For this review, take the finished solid that the model builds, in its own axes (mm). Give positions to 0.01 mm unless a question says otherwise; leave off trailing zeros. Loops run counter-clockwise (first coordinate to the right, second up) from the corner with the lowest first, then second, coordinate; pieces in that order, holes last.
```python
from build123d import *

# Parameters (mm, degrees)
SKETCH1_R           = 1.5
BOSS_EXTRUDE1_DEPTH = 3
BOSS_EXTRUDE2_DEPTH = 3
LPATTERN1_COUNT     = 2
LPATTERN1_PITCH     = 25
BOSS_EXTRUDE3_DEPTH = 3
SKETCH1_4_R         = 1.5
BOSS_EXTRUDE4_DEPTH = 15


with BuildPart() as part:
    # Sketch1 → Boss-Extrude1 (new body)
    with BuildSketch(Plane(origin=(0, 0, 0), x_dir=(1, 0, 0), z_dir=(0, 1, 0))):
        Polygon((0, 53.3), (57.3, 53.3), (57.3, 0), (0, 0), (0, 51.3), align=None)
        with Locations(Location((3, 3, 0), (0, 0, 270))):
            Circle(SKETCH1_R, mode=Mode.SUBTRACT)
        with Locations(Location((54.4, 8, 0), (0, 0, 270))):
            Circle(SKETCH1_R, mode=Mode.SUBTRACT)
        with Locations(Location((54.4, 35.5, 0), (0, 0, 270))):
            Circle(SKETCH1_R, mode=Mode.SUBTRACT)
        with Locations(Location((4, 50.8, 0), (0, 0, 270))):
            Circle(SKETCH1_R, mode=Mode.SUBTRACT)
        with BuildLine():
            Line((6.5, 3), (54.4, 3))
            Line((54.4, 3), (54.4, 4.5))
            ThreePointArc((54.4, 4.5), (50.9, 8), (54.4, 11.5))
            Line((54.4, 11.5), (54.4, 32))
            ThreePointArc((54.4, 32), (50.9, 35.5), (54.4, 39))
            Line((54.4, 39), (54.4, 50.8))
            Line((54.4, 50.8), (7.5, 50.8))
            ThreePointArc((7.5, 50.8), (6.006240265, 47.93207392), (2.8, 47.512143555))
            Line((2.8, 47.512143555), (3, 6.5))
            ThreePointArc((3, 6.5), (5.474873734, 5.474873734), (6.5, 3))
        make_face(mode=Mode.SUBTRACT)
    extrude(amount=BOSS_EXTRUDE1_DEPTH)

    # Sketch1_3 → Boss-Extrude2 (add)
    with BuildSketch(Plane(origin=(0, 0, 0), x_dir=(1, 0, 0), z_dir=(0, 1, 0))):
        with BuildLine():
            Line((-4.2, 49.3), (0, 49.3))
            Line((0, 49.3), (0, 51.3))
            Line((0, 51.3), (0, 53.3))
            Line((0, 53.3), (-4.2, 53.3))
            Line((-4.2, 53.3), (-4.2, 56.3))
            Line((-4.2, 56.3), (-5.2, 56.3))
            ThreePointArc((-5.2, 56.3), (-6.614213562, 55.714213562), (-7.2, 54.3))
            Line((-7.2, 54.3), (-7.2, 48.3))
            ThreePointArc((-7.2, 48.3), (-6.614213562, 46.885786438), (-5.2, 46.3))
            Line((-5.2, 46.3), (-4.2, 46.3))
            Line((-4.2, 46.3), (-4.2, 49.3))
        make_face()
    boss_extrude2 = extrude(amount=BOSS_EXTRUDE2_DEPTH)

    # LPattern1: Boss-Extrude2 ×2
    with Locations(*[(0, 0, i * LPATTERN1_PITCH) for i in range(1, LPATTERN1_COUNT)]):
        add(boss_extrude2)

    # Sketch2 → Boss-Extrude3 (add)
    with BuildSketch(Plane.XY):
        Polygon((0, 0), (0, 15.203282646), (10.735764429, 0), align=None)
    extrude(amount=BOSS_EXTRUDE3_DEPTH)

    # Sketch1_4 → Boss-Extrude4 (add)
    with BuildSketch(Plane(origin=(0, 0, 0), x_dir=(1, 0, 0), z_dir=(0, 1, 0))):
        with Locations(Location((54.4, 8, 0), (0, 0, 270))):
            Circle(SKETCH1_4_R)
        with Locations(Location((54.4, 35.5, 0), (0, 0, 270))):
            Circle(SKETCH1_4_R)
        with Locations(Location((4, 50.8, 0), (0, 0, 270))):
            Circle(SKETCH1_4_R)
        with Locations(Location((3, 3, 0), (0, 0, 270))):
            Circle(SKETCH1_4_R)
    extrude(amount=BOSS_EXTRUDE4_DEPTH)


solid = part.part
```
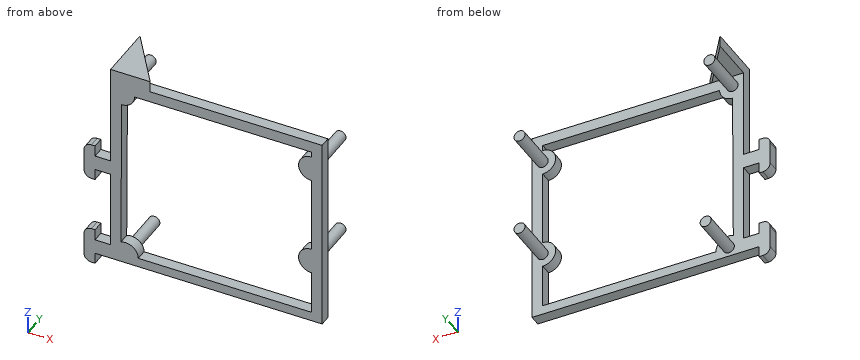
Item 1: Take a section at B-B on y = 3.75. Give the boundary of the cut face in (x, z), and give its area (3 significant figures).
Answer:
outline: (0, 0) - (8.09, 0) - (8.09, 3) - (0, 3) - close; circle Ø3 at (3, -3); circle Ø3 at (4, -50.8); circle Ø3 at (54.4, -35.5); circle Ø3 at (54.4, -8)
area: 52.5 mm2
Item 2: For L1, parallel to Y at x = 2, z = -39; L2, parallel to Z at x = 53.5, y = 5; L3, parallel to X at y = 2, z = -38, list the stretches that pass through material, from the lowest coordinate up.
Answer:
L1: y = 0 to 3
L2: z = -36.7 to -34.3, -9.2 to -6.8
L3: x = 0 to 2.85, 51.95 to 57.3
Item 3: Take a section at D-D on z = -35.5. Give the boundary of the cut face in (x, y).
Answer:
outline: (0, 0) - (2.86, 0) - (2.86, 3) - (0, 3) - close; (50.9, 0) - (57.3, 0) - (57.3, 3) - (55.9, 3) - (55.9, 15) - (52.9, 15) - (52.9, 3) - (50.9, 3) - close
Item 4: Take a section at C-C on z = -16.5. Give the boundary of the cut face in (x, y), and give its area (3 significant figures).
Answer:
outline: (0, 0) - (2.95, 0) - (2.95, 3) - (0, 3) - close; (54.4, 0) - (57.3, 0) - (57.3, 3) - (54.4, 3) - close
area: 17.6 mm2
Item 5: Clearance check with flat-ended pins moving along their axes: pin 1 Ø2.5 at (x, y) = (33.5, 2) entering from -Z; pin 2 Ø1.5 at (x, y) = (37.5, 2) entering from +Z; pin 3 Ø1 at (y, z) = (2, -21) entering from -X. State where each tip first meets the part, or that it passes through.
Answer:
pin 1: stops at z = -53.3
pin 2: stops at z = 0
pin 3: stops at x = -6.07
Item 6: Take a section at A-A on x = 44. Give the boundary of the cut face in (y, z).
Answer:
outline: (0, -53.3) - (3, -53.3) - (3, -50.8) - (0, -50.8) - close; (0, -3) - (3, -3) - (3, 0) - (0, 0) - close
